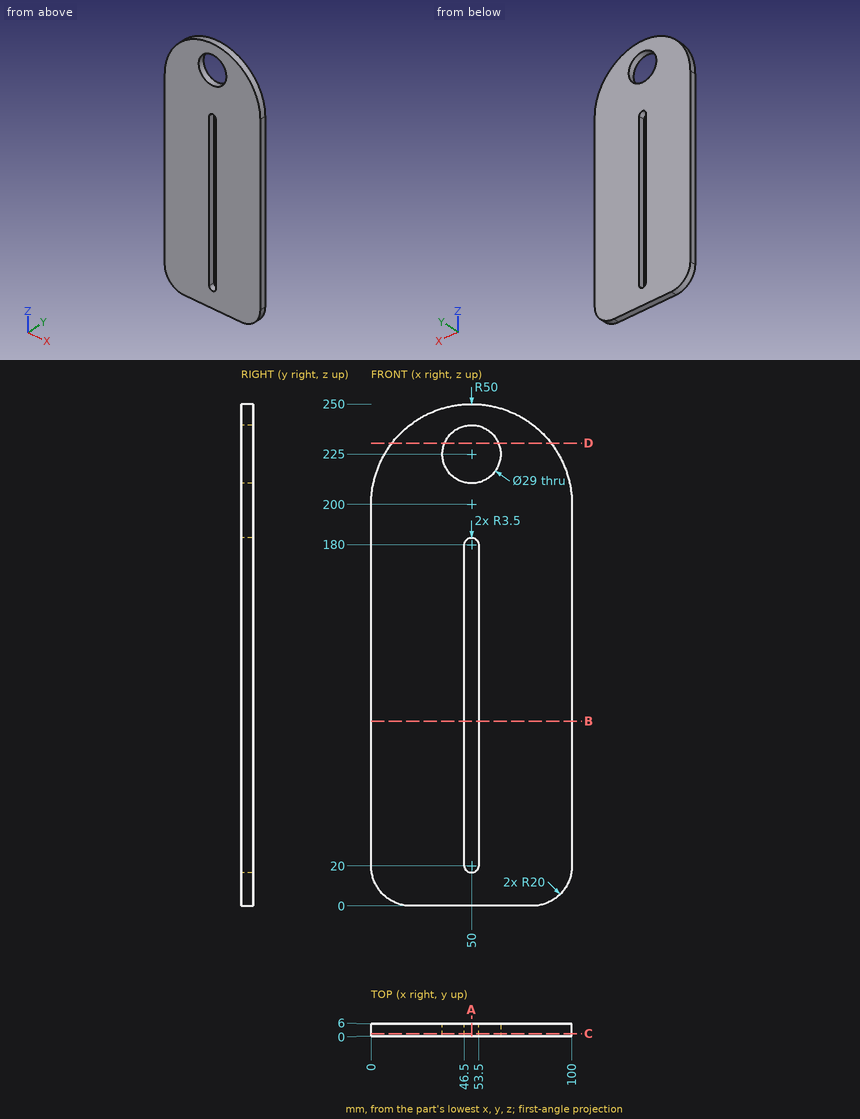
For this review, use the dimensioned drawing (mm, ordinates from the lowest corner) and the shaded views. Give positions to 0.01 mm unless a question says otherwise; leave off trailing zeros. Loops run counter-clockwise (first coordinate to the right, second up) from the corner with the lowest first, then second, coordinate; pieces in that order, holes last. Notation, with made-up numbers: (49.25, -30) -> (87.25, -30) arc R24 ccw to (87.25, -15) -> close; hole circle Ø11 at (-1.75, 60). An arc over 180 degrees is marked (long way). One line per question, with ' | ' between items. Start each with the question number.
(1) We need section C-C (y = 1.2). State the section outline as (x, z) points.
(2) We need section B-B (z = 92). State the section outline as (x, y) points, and give its area (3 significant figures).
(3) For line 1 (Z direction, x = 50, y = 2.65); line 2 (X direction, y = 5.65, z = 99); line 3 (X direction, y = 3.4, z = 225.5), list the stretches that pass through material, from the lowest coordinate up.
(4) Insertion check: P1, Ø2, axis at x = 23.5, y = 2, coming from the +Z side. The pin has a flat end and moves straight along its axis. Give the tip position at first contact, or say it passes through.
(5) We need section D-D (z = 230.5). State the section outline as (x, y) points.
(6) We need section A-A (x = 50). State the section outline as (y, z) points, and give its area (3 significant figures).
The answers:
1) outline: (0, 20) arc R20 ccw to (20, 0) -> (80, 0) arc R20 ccw to (100, 20) -> (100, 200) arc R50 ccw to (0, 200) -> close; hole circle Ø29 at (50, 225); hole (46.5, 20) arc R3.5 ccw to (53.5, 20) -> (53.5, 180) arc R3.5 ccw to (46.5, 180) -> close
2) outline: (0, 0) -> (46.5, 0) -> (46.5, 6) -> (0, 6) -> close; (53.5, 0) -> (100, 0) -> (100, 6) -> (53.5, 6) -> close | area: 558 mm^2
3) line 1: z = 0 to 16.5, 183.5 to 210.5, 239.5 to 250 | line 2: x = 0 to 46.5, 53.5 to 100 | line 3: x = 6.99 to 35.51, 64.49 to 93.01
4) P1: stops at z = 243.01
5) outline: (10.38, 0) -> (36.58, 0) -> (36.58, 6) -> (10.38, 6) -> close; (63.42, 0) -> (89.62, 0) -> (89.62, 6) -> (63.42, 6) -> close
6) outline: (0, 0) -> (6, 0) -> (6, 16.5) -> (0, 16.5) -> close; (0, 183.5) -> (6, 183.5) -> (6, 210.5) -> (0, 210.5) -> close; (0, 239.5) -> (6, 239.5) -> (6, 250) -> (0, 250) -> close | area: 324 mm^2
